```python
from build123d import *

# Parameters (mm, degrees)
SKETCH2_W                          = 127
SKETCH2_H                          = 114.3
BOSS_EXTRUDE1_DEPTH                = 1
FILLET1_R                          = 10
F_4_4_4_4_DIAMETER_HOLE1_D         = 4.4
CUT_EXTRUDE1_DEPTH                 = 171.863951728
CUT_EXTRUDE1_DEPTH_BACK            = 171.863951728
SKETCH5_W                          = 43
SKETCH5_H                          = 12.7
CUT_EXTRUDE2_DEPTH                 = 171.863951728
CUT_EXTRUDE2_DEPTH_BACK            = 171.863951728
SKETCH6_W                          = 81
SKETCH6_H                          = 5
F_3_9_3_9_DIAMETER_HOLE1_OUTLINE_R = 1.95
F_3_9_3_9_DIAMETER_HOLE1_DEPTH     = 1
FILLET2_R                          = 1


# Read off the part's stored shape, not the designer's step: Ø3.9 (3.9) Diameter Hole1
with BuildPart() as part:
    # Sketch2 → Boss-Extrude1 (new body)
    with BuildSketch(Plane(origin=(0, 0, 0), x_dir=(1, 0, 0), z_dir=(0, 1, 0))):
        with Locations((63.5, 57.15)):
            Rectangle(SKETCH2_W, SKETCH2_H)
    extrude(amount=BOSS_EXTRUDE1_DEPTH)

    # Fillet1
    fillet1_edges = [part.edges().sort_by_distance(p)[0] for p in [
        (0, 0.5, 0),
        (0, 0.5, -114.3),
        (127, 0.5, -114.3),
        (127, 0.5, 0),
    ]]
    fillet(fillet1_edges, radius=FILLET1_R)

    # Ø4.4 (4.4) Diameter Hole1 (through all)
    with Locations(Plane(origin=(0, 1, 0), x_dir=(1, 0, 0), z_dir=(0, 1, 0))):
        with Locations((10, 104.3), (117, 104.3), (10, 10), (117, 10)):
            Hole(F_4_4_4_4_DIAMETER_HOLE1_D / 2)

    # Sketch5 → Cut-Extrude1 (cut, two sides: drawn at the far end of the back side and taken through both)
    with BuildSketch(Plane(origin=(0, 1, 0), x_dir=(1, 0, 0), z_dir=(0, 1, 0)).offset(-CUT_EXTRUDE1_DEPTH_BACK)):
        with Locations((90, 68.5)):
            Rectangle(SKETCH5_W, SKETCH5_H)
        with Locations((37, 68.5)):
            Rectangle(SKETCH5_W, SKETCH5_H)
        with Locations((37, 91.2)):
            Rectangle(SKETCH5_W, SKETCH5_H)
        with Locations((90, 91.2)):
            Rectangle(SKETCH5_W, SKETCH5_H)
        with Locations((90, 23.1)):
            Rectangle(SKETCH5_W, SKETCH5_H)
        with Locations((90, 45.8)):
            Rectangle(SKETCH5_W, SKETCH5_H)
        with Locations((37, 45.8)):
            Rectangle(SKETCH5_W, SKETCH5_H)
        with Locations((37, 23.1)):
            Rectangle(SKETCH5_W, SKETCH5_H)
    extrude(amount=CUT_EXTRUDE1_DEPTH + CUT_EXTRUDE1_DEPTH_BACK, mode=Mode.SUBTRACT)

    # Sketch6 → Cut-Extrude2 (cut, two sides: drawn at the far end of the back side and taken through both)
    with BuildSketch(Plane(origin=(0, 1, 0), x_dir=(1, 0, 0), z_dir=(0, 1, 0)).offset(-CUT_EXTRUDE2_DEPTH_BACK)):
        with Locations((63.5, 106.8)):
            Rectangle(SKETCH6_W, SKETCH6_H)
        with Locations((63.5, 7.5)):
            Rectangle(SKETCH6_W, SKETCH6_H)
    extrude(amount=CUT_EXTRUDE2_DEPTH + CUT_EXTRUDE2_DEPTH_BACK, mode=Mode.SUBTRACT)

    # Ø3.9 (3.9) Diameter Hole1 outline → Ø3.9 (3.9) Diameter Hole1 (cut)
    with BuildSketch(Plane(origin=(0, 0, 0), x_dir=(1, 0, 0), z_dir=(0, 1, 0))):
        with Locations((117, 34.45)):
            Circle(F_3_9_3_9_DIAMETER_HOLE1_OUTLINE_R)
        with Locations((103.625, 34.45)):
            Circle(F_3_9_3_9_DIAMETER_HOLE1_OUTLINE_R)
        with Locations((76.625, 34.45)):
            Circle(F_3_9_3_9_DIAMETER_HOLE1_OUTLINE_R)
        with Locations((90, 34.45)):
            Circle(F_3_9_3_9_DIAMETER_HOLE1_OUTLINE_R)
        with Locations((50.125, 34.45)):
            Circle(F_3_9_3_9_DIAMETER_HOLE1_OUTLINE_R)
        with Locations((63.5, 34.45)):
            Circle(F_3_9_3_9_DIAMETER_HOLE1_OUTLINE_R)
        with Locations((23.625, 34.45)):
            Circle(F_3_9_3_9_DIAMETER_HOLE1_OUTLINE_R)
        with Locations((10, 34.45)):
            Circle(F_3_9_3_9_DIAMETER_HOLE1_OUTLINE_R)
        with Locations((37, 34.45)):
            Circle(F_3_9_3_9_DIAMETER_HOLE1_OUTLINE_R)
        with Locations((10, 57.15)):
            Circle(F_3_9_3_9_DIAMETER_HOLE1_OUTLINE_R)
        with Locations((23.625, 57.15)):
            Circle(F_3_9_3_9_DIAMETER_HOLE1_OUTLINE_R)
        with Locations((37, 57.15)):
            Circle(F_3_9_3_9_DIAMETER_HOLE1_OUTLINE_R)
        with Locations((50.125, 57.15)):
            Circle(F_3_9_3_9_DIAMETER_HOLE1_OUTLINE_R)
        with Locations((63.5, 57.15)):
            Circle(F_3_9_3_9_DIAMETER_HOLE1_OUTLINE_R)
        with Locations((76.625, 57.15)):
            Circle(F_3_9_3_9_DIAMETER_HOLE1_OUTLINE_R)
        with Locations((90, 57.15)):
            Circle(F_3_9_3_9_DIAMETER_HOLE1_OUTLINE_R)
        with Locations((103.625, 57.15)):
            Circle(F_3_9_3_9_DIAMETER_HOLE1_OUTLINE_R)
        with Locations((117, 79.85)):
            Circle(F_3_9_3_9_DIAMETER_HOLE1_OUTLINE_R)
        with Locations((103.625, 79.85)):
            Circle(F_3_9_3_9_DIAMETER_HOLE1_OUTLINE_R)
        with Locations((117, 57.15)):
            Circle(F_3_9_3_9_DIAMETER_HOLE1_OUTLINE_R)
        with Locations((76.625, 79.85)):
            Circle(F_3_9_3_9_DIAMETER_HOLE1_OUTLINE_R)
        with Locations((90, 79.85)):
            Circle(F_3_9_3_9_DIAMETER_HOLE1_OUTLINE_R)
        with Locations((50.125, 79.85)):
            Circle(F_3_9_3_9_DIAMETER_HOLE1_OUTLINE_R)
        with Locations((63.5, 79.85)):
            Circle(F_3_9_3_9_DIAMETER_HOLE1_OUTLINE_R)
        with Locations((23.625, 79.85)):
            Circle(F_3_9_3_9_DIAMETER_HOLE1_OUTLINE_R)
        with Locations((37, 79.85)):
            Circle(F_3_9_3_9_DIAMETER_HOLE1_OUTLINE_R)
        with Locations((10, 79.85)):
            Circle(F_3_9_3_9_DIAMETER_HOLE1_OUTLINE_R)
    extrude(amount=F_3_9_3_9_DIAMETER_HOLE1_DEPTH, mode=Mode.SUBTRACT)

    # Fillet2
    fillet2_edges = [part.edges().sort_by_distance(p)[0] for p in [
        (111.5, 0.5, -97.55),
        (111.5, 0.5, -84.85),
        (68.5, 0.5, -84.85),
        (68.5, 0.5, -97.55),
        (68.5, 0.5, -62.15),
        (68.5, 0.5, -74.85),
        (111.5, 0.5, -74.85),
        (111.5, 0.5, -62.15),
        (15.5, 0.5, -84.85),
        (15.5, 0.5, -97.55),
        (58.5, 0.5, -97.55),
        (58.5, 0.5, -84.85),
        (68.5, 0.5, -52.15),
        (111.5, 0.5, -52.15),
        (111.5, 0.5, -39.45),
        (68.5, 0.5, -39.45),
        (58.5, 0.5, -52.15),
        (58.5, 0.5, -39.45),
        (15.5, 0.5, -39.45),
        (15.5, 0.5, -52.15),
        (15.5, 0.5, -16.75),
        (15.5, 0.5, -29.45),
        (58.5, 0.5, -29.45),
        (58.5, 0.5, -16.75),
        (58.5, 0.5, -74.85),
        (58.5, 0.5, -62.15),
        (15.5, 0.5, -62.15),
        (15.5, 0.5, -74.85),
        (23, 0.5, -104.3),
        (23, 0.5, -109.3),
        (104, 0.5, -109.3),
        (104, 0.5, -104.3),
        (23, 0.5, -5),
        (23, 0.5, -10),
        (104, 0.5, -10),
        (104, 0.5, -5),
        (68.5, 0.5, -29.45),
        (111.5, 0.5, -29.45),
        (111.5, 0.5, -16.75),
        (68.5, 0.5, -16.75),
    ]]
    fillet(fillet2_edges, radius=FILLET2_R)


solid = part.part
```
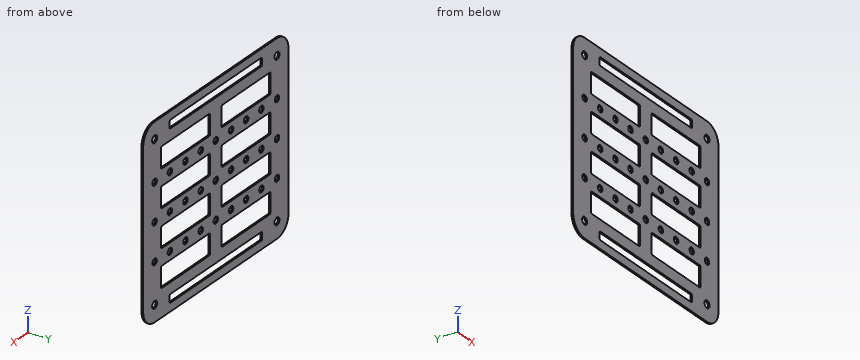
Geometry check sheet. Reference: the model listing, model coordinates, mm. Give positions to 0.01 mm unless a question says otherwise; leave off trailing zeros. Order: outer loops, then holes, each group sorted by start corner. A loop starts at its lowest first (then second) coordinate and runs counter-clockwise, first axis right, second up. Notation, with made-up numbers: (-5.75, 32.25) - (37.25, 32.25) arc R6 cw to (37.25, 37.25) - close; hole circle Ø3 at (44, 85.25). An arc over 180 degrees is marked (long way). Write item = value, one per line. Start each with the question number.
1) Gauge pin test, flat end, axial feed: pin 1 Ø3 at (x, z) = (23.625, -57.15) entering from -Y. Record the tip position at first contact, or that the pin passes through.
2) Section check B-B (x = 90). Count the separate pieces of the cut face and the enclosed holes in it, then the cut area to 3 significant figures.
3) Scan lines: L1, parallel to Z at x = 117, y = 0.2; L2, parallel to Z at x = 61, y = 0.2; L3, parallel to X at y = 0.3, z = -46.5. Record each from-to range of solid material in increasing order.
4) Section check A-A (x = 63.5). Enter the section's corners in (y, z).
Geometry check:
q1.pin_1 = through
q2.separate_pieces = 10
q2.enclosed_holes = 0
q2.area = 41.8 mm2
q3.L1 = -114.3 to -106.5, -102.1 to -81.8, -77.9 to -59.1, -55.2 to -36.4, -32.5 to -12.2, -7.8 to 0
q3.L2 = -114.3 to -109.3, -104.3 to -10, -5 to 0
q3.L3 = 0 to 15.5, 58.5 to 68.5, 111.5 to 127
q4.outline = (0, -114.3) - (1, -114.3) - (1, -109.3) - (0, -109.3) - close; (0, -104.3) - (1, -104.3) - (1, -81.8) - (0, -81.8) - close; (0, -77.9) - (1, -77.9) - (1, -59.1) - (0, -59.1) - close; (0, -55.2) - (1, -55.2) - (1, -36.4) - (0, -36.4) - close; (0, -32.5) - (1, -32.5) - (1, -10) - (0, -10) - close; (0, -5) - (1, -5) - (1, 0) - (0, 0) - close
